```python
from build123d import *

# Parameters (mm, degrees)
CROQUIS1_W               = 52.6
CROQUIS1_H               = 45
CROQUIS1_R               = 5.4
CROQUIS1_R_2             = 2
SALIENTE_EXTRUIR1_DEPTH  = 5
CROQUIS2_W               = 5
CROQUIS2_H               = 8
SALIENTE_EXTRUIR2_DEPTH  = 5
REDONDEO1_R              = 0.5
REDONDEO1_OF_SIMETR_A1_R = 0.5
CROQUIS3_W               = 20
CROQUIS3_H               = 8
CORTAR_EXTRUIR1_DEPTH    = 5
REDONDEO2_R              = 2
CROQUIS4_W               = 52.6
CROQUIS4_H               = 0.6
CORTAR_EXTRUIR2_DEPTH    = 5


with BuildPart() as part:
    # Croquis1 → Saliente-Extruir1 (new body)
    with BuildSketch(Plane.XY):
        Rectangle(CROQUIS1_W, CROQUIS1_H)
        with Locations((0, -1.5)):
            Circle(CROQUIS1_R, mode=Mode.SUBTRACT)
        with Locations((-5.656854249, 4.156854249)):
            Circle(CROQUIS1_R_2, mode=Mode.SUBTRACT)
        with Locations((5.656854249, 4.156854249)):
            Circle(CROQUIS1_R_2, mode=Mode.SUBTRACT)
        with Locations((5.656854249, -7.156854249)):
            Circle(CROQUIS1_R_2, mode=Mode.SUBTRACT)
        with Locations((-5.656854249, -7.156854249)):
            Circle(CROQUIS1_R_2, mode=Mode.SUBTRACT)
    extrude(amount=SALIENTE_EXTRUIR1_DEPTH)

    # Croquis2 → Saliente-Extruir2 (add)
    with BuildSketch(Plane.ZY.offset(26.3)):
        with Locations((2.5, 15)):
            Rectangle(CROQUIS2_W, CROQUIS2_H)
        with Locations((2.5, -15)):
            Rectangle(CROQUIS2_W, CROQUIS2_H)
    saliente_extruir2 = extrude(amount=SALIENTE_EXTRUIR2_DEPTH)

    # Redondeo1
    redondeo1_edges = [part.edges().sort_by_distance(p)[0] for p in [
        (-28.8, 19, 0),
        (-28.8, 11, 0),
        (-28.8, 11, 5),
        (-28.8, 19, 5),
        (-31.3, 15, 0),
        (-31.3, 11, 2.5),
        (-31.3, 15, 5),
        (-31.3, 19, 2.5),
        (-28.8, -19, 0),
        (-28.8, -19, 5),
        (-28.8, -11, 5),
        (-28.8, -11, 0),
        (-31.3, -19, 2.5),
        (-31.3, -15, 5),
        (-31.3, -11, 2.5),
        (-31.3, -15, 0),
    ]]
    fillet(redondeo1_edges, radius=REDONDEO1_R)

    # Simetría1: Saliente-Extruir2 across plane
    add(saliente_extruir2.mirror(Plane(origin=(0, 0, 0), x_dir=(0, 0, 1), z_dir=(1, 0, 0))))

    # Redondeo1 of Simetría1
    redondeo1_of_simetr_a1_edges = [part.edges().sort_by_distance(p)[0] for p in [
        (28.8, 19, 0),
        (28.8, 11, 0),
        (28.8, 11, 5),
        (28.8, 19, 5),
        (31.3, 15, 0),
        (31.3, 11, 2.5),
        (31.3, 15, 5),
        (31.3, 19, 2.5),
        (28.8, -19, 0),
        (28.8, -19, 5),
        (28.8, -11, 5),
        (28.8, -11, 0),
        (31.3, -19, 2.5),
        (31.3, -15, 5),
        (31.3, -11, 2.5),
        (31.3, -15, 0),
    ]]
    fillet(redondeo1_of_simetr_a1_edges, radius=REDONDEO1_OF_SIMETR_A1_R)

    # Croquis3 → Cortar-Extruir1 (cut)
    with BuildSketch(Plane.XY.offset(5)):
        with Locations((0, 18.5)):
            Rectangle(CROQUIS3_W, CROQUIS3_H)
    extrude(amount=-CORTAR_EXTRUIR1_DEPTH, mode=Mode.SUBTRACT)

    # Redondeo2
    redondeo2_edges = [part.edges().sort_by_distance(p)[0] for p in [
        (-10, 14.5, 2.5),
        (-10, 22.5, 2.5),
        (10, 22.5, 2.5),
        (10, 14.5, 2.5),
    ]]
    fillet(redondeo2_edges, radius=REDONDEO2_R)

    # Croquis4 → Cortar-Extruir2 (cut)
    with BuildSketch(Plane.XY.offset(5)):
        with Locations((0, -22.2)):
            Rectangle(CROQUIS4_W, CROQUIS4_H)
    extrude(amount=-CORTAR_EXTRUIR2_DEPTH, mode=Mode.SUBTRACT)


solid = part.part
```
Design review of the part built by this model. Coordinates are the model's own, in mm. A direction names the side the tool comes from. Round coordinates to 2 decimals unless told otherwise and drop trailing zeros. Order: outer loops, then holes, each group sorted by start corner. A loop starts at its lowest first (then second) coordinate and runs counter-clockwise, first axis right, second up. Notation, with made-up numbers: (74, 57) - (132, 57) arc R21 ccw to (132, 87) - close; hole circle Ø4 at (34, 76). An arc over 180 degrees is marked (long way). One line per question, with ' | ' between items.
Item 1: Draft analysis for pull direction X (two halves, no side actions). For faces 4 (the face through (-10.6, 21.93, 2.46)), 5 (the face through (29, -19, 2)), 6 (the face through (-31.3, -15, 2)), state which applies: +X half, -X half, draft (parallel to the pull), parting line (faces both ways), or undercut.
Checks:
face 4: undercut | face 5: draft | face 6: -X half
Item 2: Machinability: for faces 1 (the face through (9.4, 15.07, 2.46)), 2 (the face through (-29, 19, 2)), 3 (the face through (-29, -19, 2)), which of the approach directions +Z, -Z, +X, -X, +Y, -Y give a long, thin tool a straight path to every point of the face, cutting with its end or side? Answer none if there is none.
Checks:
face 1: +Z, -Z, +Y | face 2: +Z, -Z, -X, +Y | face 3: +Z, -Z, -X, -Y
Item 3: Take a section at D-D, the plane z = 3.3. Give the number of separate pieces and of enclosed holes in the cut face, then the cut area to 3 significant figures.
Checks:
separate pieces: 1 | enclosed holes: 5 | area: 2,190 mm²
Item 4: Take a section at C-C, the plane y = -8.5. Write out the cut boundary in (x, z), then the cut area to 3 significant figures.
Checks:
outline: (-26.3, 0) - (-7.14, 0) - (-7.14, 5) - (-26.3, 5) - close; (-4.17, 0) - (4.17, 0) - (4.17, 5) - (-4.17, 5) - close; (7.14, 0) - (26.3, 0) - (26.3, 5) - (7.14, 5) - close | area: 233 mm²
Item 5: Wall thickness on line 1 (Y direction, x = -6.5, z = 1.75); line 2 (X direction, y = -7, z = 0.95); line 3 (Y direction, x = -7, z = 1.6): over which ranges is each line inside the solid? List them lowest first. Write a range as [from, to].
Checks:
line 1: [-21.9, -8.97], [-5.34, 2.34], [5.97, 14.5] | line 2: [-26.3, -7.65], [-3.66, 3.66], [7.65, 26.3] | line 3: [-21.9, -8.64], [-5.67, 2.67], [5.64, 14.5]
Item 6: For P1, Ø2, axis at x = 29.5, z = 3.5, coming from the +Y side; P2, Ø5, axis at x = 5.66, y = 4.16, coming from the +Z side; P3, Ø1, axis at y = -21, z = 2, coming from the +X side; P4, Ø1.2, axis at x = -29, z = 3, coming from the -Y side, all flat-tipped, find the tip position at first contact; note any pin that passes through.
Checks:
P1: y = 19 | P2: z = 5 | P3: x = 26.3 | P4: y = -19
Item 7: Take a section at B-B, the plane x = 0. Write out the cut boundary in (y, z).
Checks:
outline: (-21.9, 0) - (-6.9, 0) - (-6.9, 5) - (-21.9, 5) - close; (3.9, 0) - (14.5, 0) - (14.5, 5) - (3.9, 5) - close
Item 8: Take a section at A-A, the plane y = -1.5. Write out the cut boundary in (x, z), then the cut area to 3 significant figures.
Checks:
outline: (-26.3, 0) - (-5.4, 0) - (-5.4, 5) - (-26.3, 5) - close; (5.4, 0) - (26.3, 0) - (26.3, 5) - (5.4, 5) - close | area: 209 mm²
